```python
from build123d import *

# Parameters (mm, degrees)
SKETCH1_W           = 1000
SKETCH1_H           = 300
BOSS_EXTRUDE1_DEPTH = 500
SHELL1_T            = -40
SKETCH3_W           = 940
SKETCH3_H           = 440
CUT_EXTRUDE1_DEPTH  = 240
SKETCH4_W           = 940
SKETCH4_H           = 20
BOSS_EXTRUDE2_DEPTH = 240
FILLET1_R           = 2


with BuildPart() as part:
    # Sketch1 → Boss-Extrude1 (new body)
    with BuildSketch(Plane(origin=(0, 0, 0), x_dir=(0, 1, 0), z_dir=(0, 0, 1))):
        with Locations((0, -150)):
            Rectangle(SKETCH1_W, SKETCH1_H)
    extrude(amount=BOSS_EXTRUDE1_DEPTH)

    # Shell1
    shell1_openings = [part.faces().sort_by_distance(p)[0] for p in [
        (300, 0, 250),
    ]]
    offset(amount=SHELL1_T, openings=shell1_openings, kind=Kind.INTERSECTION)

    # Sketch3 → Cut-Extrude1 (cut)
    with BuildSketch(Plane.YZ.offset(40)):
        with Locations((0, 250)):
            Rectangle(SKETCH3_W, SKETCH3_H)
    extrude(amount=CUT_EXTRUDE1_DEPTH, mode=Mode.SUBTRACT)

    # Sketch4 → Boss-Extrude2 (add)
    with BuildSketch(Plane.YZ.offset(40)):
        with Locations((0, 250)):
            Rectangle(SKETCH4_W, SKETCH4_H)
    extrude(amount=BOSS_EXTRUDE2_DEPTH)

    # Fillet1
    fillet1_edges = [part.edges().sort_by_distance(p)[0] for p in [
        (150, 500, 500),
        (300, 0, 40),
        (300, -460, 250),
        (0, 0, 500),
        (300, 460, 250),
        (300, 0, 460),
        (150, -500, 500),
        (0, 0, 0),
        (150, 500, 0),
        (280, 0, 240),
        (280, 0, 260),
        (300, 0, 0),
        (150, -500, 0),
        (0, -500, 250),
        (0, 500, 250),
        (300, 500, 250),
        (300, -500, 250),
        (300, 0, 500),
    ]]
    fillet(fillet1_edges, radius=FILLET1_R)


solid = part.part
```
Work out the finished part from the listing and answer in its coordinate system (mm). A direction names the side the tool comes from. Coordinates: 2 decimals unless noted, no trailing zeros. Write each loop counter-clockwise with the first axis right and the second up, starting at its lowest first coordinate (ties: lowest second). Pieces come first, ordered by that corner, then holes.
Q1. Determine the mould class of faces 4 (the face through (290, -460, 247)), 5 (the face through (152, 500, 247)), 6 (the face through (148, -7, 0)) for opening direction Z: released by +Z, released by -Z, zero draft, split by the parting line, or undercut.
Q2. Find the intervals of material crossed by line 1 (Z direction, x = 177, y = 202.5); line 2 (Y direction, x = 229, z = 210.5); line 3 (X direction, y = 35, z = 274), in increasing order.
Q3. Which of the six approach directions +Z, -Z, +X, -X, +Y, -Y give full straight-line access (tool end or side, diameter ignored) to faces 1 (the face through (289, -6, 40)), 2 (the face through (280, -2, 34)), 3 (the face through (0, -7, 247))?
Q4. A cutting plane is placed at A-A, the plane z = 133. Give the vertices of the cut face in (x, y).
Q5. A cutting plane is placed at B-B, the plane x = 158. Give the vertices of the cut face in (y, z).
Q6. Each of these flat-tipped pins is pushed along its axis until it touches: pin 1 Ø10 at (y, z) = (-381, 295.5) entering from +X; pin 2 Ø17.5 at (y, z) = (55.5, 252.5) entering from +X. Where does it stop, or does it pass through?
Q7. A cutting plane is placed at C-C, the plane y = 96. Give the vertices of the cut face in (x, z), then the cut area to 3 significant figures.
Findings below:
1. face 4: undercut
1. face 5: zero draft
1. face 6: released by -Z
2. line 1: z = 0 to 30, 240 to 260, 470 to 500
2. line 2: y = -500 to -470, 470 to 500
2. line 3: x = 0 to 40
3. face 1: +X
3. face 2: none
3. face 3: +Z, -Z, -X, +Y, -Y
4. outline: (0, -498) arc R2 ccw to (2, -500) - (298, -500) arc R2 ccw to (300, -498) - (300, -462) arc R2 ccw to (298, -460) - (280, -460) - (280, -470) - (40, -470) - (40, 470) - (280, 470) - (280, 460) - (298, 460) arc R2 ccw to (300, 462) - (300, 498) arc R2 ccw to (298, 500) - (2, 500) arc R2 ccw to (0, 498) - close
5. outline: (-500, 2) arc R2 ccw to (-498, 0) - (498, 0) arc R2 ccw to (500, 2) - (500, 498) arc R2 ccw to (498, 500) - (-498, 500) arc R2 ccw to (-500, 498) - close; hole (-470, 30) - (470, 30) - (470, 240) - (-470, 240) - close; hole (-470, 260) - (470, 260) - (470, 470) - (-470, 470) - close
6. pin 1: stops at x = 40
6. pin 2: stops at x = 280
7. outline: (0, 2) arc R2 ccw to (2, 0) - (298, 0) arc R2 ccw to (300, 2) - (300, 38) arc R2 ccw to (298, 40) - (280, 40) - (280, 30) - (40, 30) - (40, 240) - (278, 240) arc R2 ccw to (280, 242) - (280, 258) arc R2 ccw to (278, 260) - (40, 260) - (40, 470) - (280, 470) - (280, 460) - (298, 460) arc R2 ccw to (300, 462) - (300, 498) arc R2 ccw to (298, 500) - (2, 500) arc R2 ccw to (0, 498) - close
7. area: 40,800 mm2
